```python
from build123d import *

# Parameters (mm, degrees)
F1_DEPTH = 70
F2_R     = 2
F3_DEPTH = 5
F4_R     = 3
F5_DEPTH = 1.25
F6_R     = 0.3


with BuildPart() as f1:
    # F0 (on Front) → F1 (new body)
    with BuildSketch(Plane.XZ):
        with BuildLine():
            Line((3.831252, 7.572499), (6.531252, 7.572499))
            ThreePointArc((6.531252, 7.572499), (0, 10), (-6.531252, 7.572499))
            Line((-6.531252, 7.572499), (-3.831252, 7.572499))
            Line((-3.831252, 7.572499), (-5.130291, 5.322499))
            Line((-5.130291, 5.322499), (-3.630291, 5.322499))
            Line((-3.630291, 5.322499), (-2.331252, 7.572499))
            Line((-2.331252, 7.572499), (0, 7.572499))
            Line((0, 7.572499), (2.331252, 7.572499))
            Line((2.331252, 7.572499), (3.630291, 5.322499))
            Line((3.630291, 5.322499), (5.130291, 5.322499))
            Line((5.130291, 5.322499), (3.831252, 7.572499))
        make_face()
    extrude(amount=-F1_DEPTH)

    # F2 (on face) → F3 (join)
    with BuildSketch(Plane(origin=(0, 0, 7.572499), x_dir=(1, 0, 0), z_dir=(0, 0, -1))):
        with Locations((0, -6)):
            Circle(F2_R)
    extrude(amount=-F3_DEPTH)

    # F4 (on face) → F5 (join)
    with BuildSketch(Plane.XY.offset(12.572499)):
        with Locations((0, 6)):
            Circle(F4_R)
    extrude(amount=F5_DEPTH)

    # F6
    f6_edges = [f1.edges().sort_by_distance(p)[0] for p in [
        (-3, 6, 13.822499),
        (-3, 6, 12.572499),
    ]]
    fillet(f6_edges, radius=F6_R)


solid = f1.part
```
Verification items for the finished model (mm, model axes). A direction names the side the tool comes from. Coordinates: 2 decimals unless noted, no trailing zeros. Write each loop counter-clockwise with the first axis right and the second up, starting at its lowest first coordinate (ties: lowest second). Pieces come first, ordered by that corner, then holes. Notation, with made-up numbers: (-5.75, -9) - (10.25, -9) arc R27 cw to (10.25, 16) - close; hole circle Ø11 at (43, 73). An arc over 180 degrees is marked (long way). One line per question, with ' | ' between items. Start each with the question number.
1. Draft check along X on faces 6 (the flat face through (0, 0, 8)), 7 (the flat face through (4.49, 34.51, 6.43)), 8 (the flat face through (-2.99, 34.51, 6.43)). Enter one of: released by +X, released by -X, zero draft, split by the parting line, or undercut.
2. Section check B-B (x = 0). Enter the section's corners in (y, z).
3. Section check D-D (z = 11). Enter the section's corners in (x, y), plus the area to 3 significant figures.
4. Gauge pin test, flat ends, axial feed: P1, Ø1.6, axis at x = 1, y = 5, coming from the -Z side; P2, Ø4, axis at x = -3.5, y = 15, coming from the +Z side; P3, Ø1, axis at x = -4.5, y = 16, coming from the +Z side. Record the tip position at first contact, or that the pin passes through.
5. Material ranges on line 1 along Z through (x, y) = (-0.25, 39); line 2 along X through (y, z) = (12.5, 6.25); line 3 along Z through (x, y) = (2, 15.5), recorded low to high.
6. Access from +Z, -Z, +X, -X, +Y, -Y to the whole of each face (thin tool, end or side, straight path). Record for faces 1 (the flat face through (0, 35, 7.572)), 2 (the flat face through (5, 35, 7.572)), 3 (the cylindrical face through (-2, 6, 11)), 4 (the cylindrical face through (-0.65, 3.07, 13.19)), 5 (the flat face through (-5, 35, 7.572)).
7. Section check A-A (y = 6). Enter the section's corners in (x, z), plus the area to 3 significant figures.
8. Section check C-C (x = 4.5). Enter the section's corners in (y, z).
Computed values:
1) face 6: zero draft | face 7: released by +X | face 8: undercut
2) outline: (0, 7.57) - (70, 7.57) - (70, 10) - (8, 10) - (8, 12.57) - (8.7, 12.57) arc R0.3 ccw to (9, 12.87) - (9, 13.52) arc R0.3 ccw to (8.7, 13.82) - (3.3, 13.82) arc R0.3 ccw to (3, 13.52) - (3, 12.87) arc R0.3 ccw to (3.3, 12.57) - (4, 12.57) - (4, 10) - (0, 10) - close
3) outline: circle Ø4 at (0, 6) | area: 12.6 mm²
4) P1: z = 7.57 | P2: z = 9.89 | P3: z = 9.17
5) line 1: 7.57 to 10 | line 2: -4.59 to -3.09, 3.09 to 4.59 | line 3: 7.57 to 9.8
6) face 1: -Z, +Y, -Y | face 2: +X, +Y, -Y | face 3: none | face 4: +Z | face 5: -X, +Y, -Y
7) outline: (-6.53, 7.57) - (-3.83, 7.57) - (-5.13, 5.32) - (-3.63, 5.32) - (-2.33, 7.57) - (2.33, 7.57) - (3.63, 5.32) - (5.13, 5.32) - (3.83, 7.57) - (6.53, 7.57) arc R10 ccw to (2, 9.8) - (2, 12.57) - (2.7, 12.57) arc R0.3 ccw to (3, 12.87) - (3, 13.52) arc R0.3 ccw to (2.7, 13.82) - (-2.7, 13.82) arc R0.3 ccw to (-3, 13.52) - (-3, 12.87) arc R0.3 ccw to (-2.7, 12.57) - (-2, 12.57) - (-2, 9.8) arc R10 ccw to start | area: 46.4 mm²
8) outline: (0, 5.32) - (70, 5.32) - (70, 6.41) - (0, 6.41) - close; (0, 7.57) - (70, 7.57) - (70, 8.93) - (0, 8.93) - close
